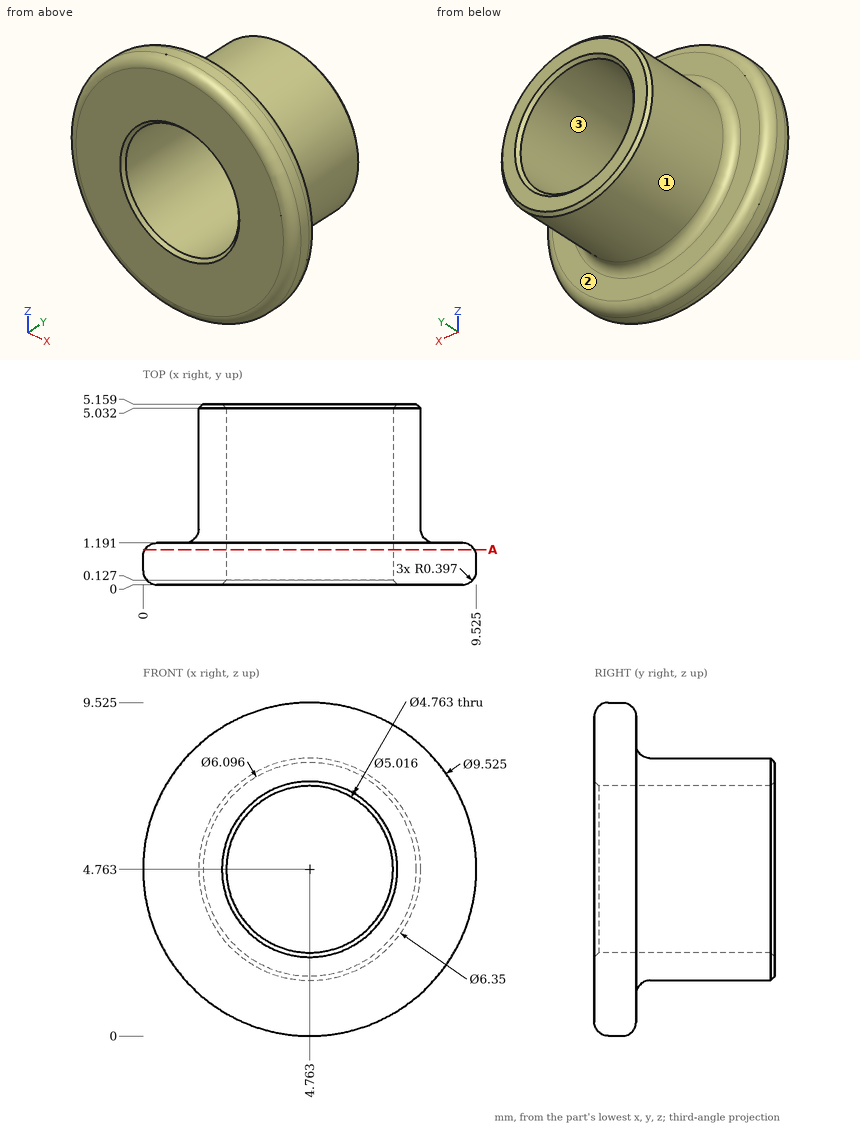
Input: dimensioned drawing with shaded views. Units: mm. Origin: part minimum x, y, z. Give positions to 0.01 mm unless a question says otherwise; leave off trailing zeros. Write each loop counter-clockwise with the first axis right and the second up, starting at its lowest first coordinate (ties: lowest second). Pieces come first, ordered by that corner, then holes. Notation, with made-up numbers: (-37, -14) - (-8, -14) arc R20 cw to (-8, -5) - close; hole circle Ø9 at (5, -22). An arc over 180 degrees is marked (long way). Write item = value, one per line. Start each with the question number.
1) Material intervals for L1, parallel to Y at x = 5.5, z = 1.25; L2, parallel to X at y = 2.55, z = 6 (1 decimal); L3, parallel to X at y = 4.45, z = 6.25 (1 decimal), sorted ascending. Write a range as [from, to].
2) Pin query (flat end, axial travel): pin 1 (1.5 mm diameter, centred on y = 1, z = 2, fed in from -X); pin 2 (1.5 mm diameter, centred on y = 2, z = 3, fed in from -X); pin 3 (1.5 mm diameter, centred on y = 2.5, z = 3.5, fed in from +X). Return the tip coordinate at first contact, or that it passes through.
3) Cut plane A-A (y = 1). Return loops of the section in (x, z) (1 decimal).
4) Draft query along X for the marked faces 1, 2 and 3. Return one class per face: pulls with the +X half, pulls with the -X half, needs draft (parallel to the pull), parting line crosses it, or undercut.
Answers follow:
q1.L1 = [0, 1.19]
q1.L2 = [1.8, 2.7], [6.8, 7.7]
q1.L3 = [2, 2.9], [6.6, 7.6]
q2.pin_1 = 0.46
q2.pin_2 = 1.75
q2.pin_3 = 7.9
q3.outline = circle Ø9.4 at (4.8, 4.8); hole circle Ø4.8 at (4.8, 4.8)
q4.face_1 = parting line crosses it
q4.face_2 = needs draft
q4.face_3 = undercut
